```python
from build123d import *

# Parameters (mm, degrees)
F0_R     = 3.175
F1_DEPTH = 3.048


with BuildPart() as f1:
    # F0 (on Front) → F1 (new body)
    with BuildSketch(Plane.XZ):
        with BuildLine():
            ThreePointArc((-7.9375, 44.45), (0, 36.5125), (7.9375, 44.45))
            ThreePointArc((7.9375, 44.45), (0, 52.3875), (-7.9375, 44.45))
        make_face()
        with Locations((0, 44.45)):
            Circle(F0_R, mode=Mode.SUBTRACT)
        with BuildLine():
            Line((8.89358, 17.782553), (7.9375, 44.45))
            ThreePointArc((7.9375, 44.45), (0, 36.5125), (-7.9375, 44.45))
            Line((-7.9375, 44.45), (-9.518884, 0.341271))
            ThreePointArc((-9.518884, 0.341271), (0.170663, 9.523471), (9.525, 0))
            ThreePointArc((9.525, 0), (6.735192, -6.735192), (0, -9.525))
            Line((0, -9.525), (61.90038, -15.794203))
            ThreePointArc((61.90038, -15.794203), (47.626332, -0.205667), (61.491711, 15.747457))
            Line((61.491711, 15.747457), (17.844427, 10.181074))
            ThreePointArc((17.844427, 10.181074), (11.692391, 12.007579), (8.89358, 17.782553))
        make_face()
        with BuildLine():
            ThreePointArc((9.525, 0), (0.170663, 9.523471), (-9.518884, 0.341271))
            ThreePointArc((-9.518884, 0.341271), (-6.854788, -6.613434), (0, -9.525))
            ThreePointArc((0, -9.525), (6.735192, -6.735192), (9.525, 0))
        make_face()
        Circle(F0_R, mode=Mode.SUBTRACT)
        with BuildLine():
            ThreePointArc((65.508289, 15.747457), (63.5, 15.875), (61.491711, 15.747457))
            ThreePointArc((61.491711, 15.747457), (47.626332, -0.205667), (61.90038, -15.794203))
            ThreePointArc((61.90038, -15.794203), (63.705667, -15.873668), (65.508289, -15.747457))
            ThreePointArc((65.508289, -15.747457), (75.414219, -10.491283), (79.375, 0))
            ThreePointArc((79.375, 0), (75.414219, 10.491283), (65.508289, 15.747457))
        make_face()
        with Locations((63.5, 0)):
            Circle(F0_R, mode=Mode.SUBTRACT)
        with BuildLine():
            Line((114.3, 9.525), (65.508289, 15.747457))
            ThreePointArc((65.508289, 15.747457), (75.414219, 10.491283), (79.375, 0))
            ThreePointArc((79.375, 0), (75.414219, -10.491283), (65.508289, -15.747457))
            Line((65.508289, -15.747457), (114.3, -9.525))
            ThreePointArc((114.3, -9.525), (104.775, 0), (114.3, 9.525))
        make_face()
        with Locations((100.0252, -3.175)):
            Circle(F0_R, mode=Mode.SUBTRACT)
        with BuildLine():
            ThreePointArc((123.825, 0), (121.035192, 6.735192), (114.3, 9.525))
            ThreePointArc((114.3, 9.525), (104.775, 0), (114.3, -9.525))
            ThreePointArc((114.3, -9.525), (121.035192, -6.735192), (123.825, 0))
        make_face()
        with Locations((114.3, 0)):
            Circle(F0_R, mode=Mode.SUBTRACT)
    extrude(amount=F1_DEPTH)


solid = f1.part
```
Input: part model. Units: mm. Frame: model coordinates. A direction names the side the tool comes from. Round coordinates to 2 decimals unless told otherwise and drop trailing zeros. Loops run counter-clockwise (first coordinate to the right, second up) from the corner with the lowest first, then second, coordinate; pieces in that order, holes last. Notation, with made-up numbers: (39.5, -13) -> (48.5, -13) arc R26 cw to (48.5, 22) -> close; hole circle Ø2 at (-27.5, 41). An arc over 180 degrees is marked (long way). One line per item, written item: value.
(1) Material intervals for line 1 (Z direction, x = 0, y = -1.75) (1 decimal); line 2 (Z direction, x = 63.5, y = -1.4) (3 decimals); line 3 (Z direction, x = 114.3, y = -1.85) (3 decimals), sorted ascending. Write a range as [from, to].
Geometry check:
line 1: [-9.5, -3.2], [3.2, 41.3], [47.6, 52.4]
line 2: [-15.875, -3.175], [3.175, 15.875]
line 3: [-9.525, -3.175], [3.175, 9.525]
(2) Section D-D (x = 15). Return the cut outline in (y, z).
Geometry check:
outline: (-3.05, -11.04) -> (0, -11.04) -> (0, 10.33) -> (-3.05, 10.33) -> close
(3) Mould query, pull axis Z, two halves, no side actions, for faces 3 (the face through (1.707, -1.503, 47.127)), 4 (the face through (63.68, -1.503, -15.874)), 5 (the face through (0.175, -1.503, 52.386)). Classes: pulls with the +Z half, pulls with the -Z half, needs draft (parallel to the pull), parting line crosses it, or undercut.
Geometry check:
face 3: undercut
face 4: pulls with the -Z half
face 5: pulls with the +Z half
(4) Section B-B (y = -0.8). Give the number of separate pieces and of enclosed holes in the cut face, plus the area to 3 significant figures.
Geometry check:
separate pieces: 1
enclosed holes: 5
area: 3,730 mm2
(5) Pin query (flat end, axial travel): pin 1 (5.5 mm diameter, centred on x = 0, z = 44.45, fed in from +Y); pin 2 (1.5 mm diameter, centred on y = -2, z = 30, fed in from -X); pin 3 (1.5 mm diameter, centred on x = 29, y = -2.5, fed in from +Z); pin 4 (1.5 mm diameter, centred on x = 52, y = -1.5, fed in from +Z). Return the tip coordinate at first contact, or that it passes through.
Geometry check:
pin 1: through
pin 2: x = -8.48
pin 3: z = 11.7
pin 4: z = 14.63
(6) Set-up query: faces 1 (the face through (39.974, -1.503, 13.003)), 2 (the face through (90.2, -1.5, 12.6)). Return all of +Z, -Z, +X, -X, +Y, -Y with unobstructed straight access to the full face (end or side cutting, diameter ignored); none if empty.
Geometry check:
face 1: +Z, +Y, -Y
face 2: +Z, +X, +Y, -Y
(7) Section C-C (z = 33). Return the cut outline in (x, y).
Geometry check:
outline: (-8.35, -3.05) -> (8.35, -3.05) -> (8.35, 0) -> (-8.35, 0) -> close
(8) Section A-A (x = 63.5). Return the cut outline in (y, z) (3 decimals), plus the area to 3 significant figures.
Geometry check:
outline: (-3.048, -15.875) -> (0, -15.875) -> (0, -3.175) -> (-3.048, -3.175) -> close; (-3.048, 3.175) -> (0, 3.175) -> (0, 15.875) -> (-3.048, 15.875) -> close
area: 77.4 mm2
